Part print with two shaded views. Sizes in mm from the minimum x, y, z corner. A direction names the side the tool comes from. Round coordinates to 2 decimals unless told otherwise and drop trailing zeros. Write each loop counter-clockwise with the first axis right and the second up, starting at its lowest first coordinate (ties: lowest second). Pieces come first, ordered by that corner, then holes. Notation, with made-up numbers: (72, 29) - (86, 29) arc R16 cw to (86, 38) - close; hole circle Ø4 at (63, 0.5). An arc over 180 degrees is marked (long way). Answer as a JSON object with one key per item and string values. Group by question number.
Item 1: Flat gauge pin, fed straight in: pin 1 (3.5 mm diameter, centred on x = 3.5, y = 4.5, fed in from -Z). Where does the tip first touch, or does it go through?
Item 2: Two-plate mould, pull along Z, no slides. Class the marked faces 4, 5 and 6: +Z half, -Z half, draft (parallel to the pull), parting line (faces both ways), or undercut.
Item 3: Which spindle directions (+Z, -Z, +X, -X, +Y, -Y) get a long thin tool onto all of the face, cutting with end or side? Do the marked faces 1, 2 and 3. Say none if no direction does.
Item 4: Slice it at C-C, the plane z = 1.25. List the corners of the cut face in (x, y).
Item 5: Slice it at D-D, the plane x = 1.75. List the corners of the cut face in (y, z), then the cut area to 3 significant figures.
Item 6: Slice it at B-B, the plane x = 9. Give the number of separate pieces and of enclosed holes in the cut face.
Item 7: Probe line 1 (Z direction, x = 4, y = 4); line 2 (Y direction, x = 8.5, z = 2) (1 decimal); line 3 (Z direction, x = 8.5, y = 10.75). List the from-to ranges inside material, lowest first. Write a range as from..to.
Item 8: Slice it at A-A, the plane z = 5.5. List the corners of the cut face in (x, y).
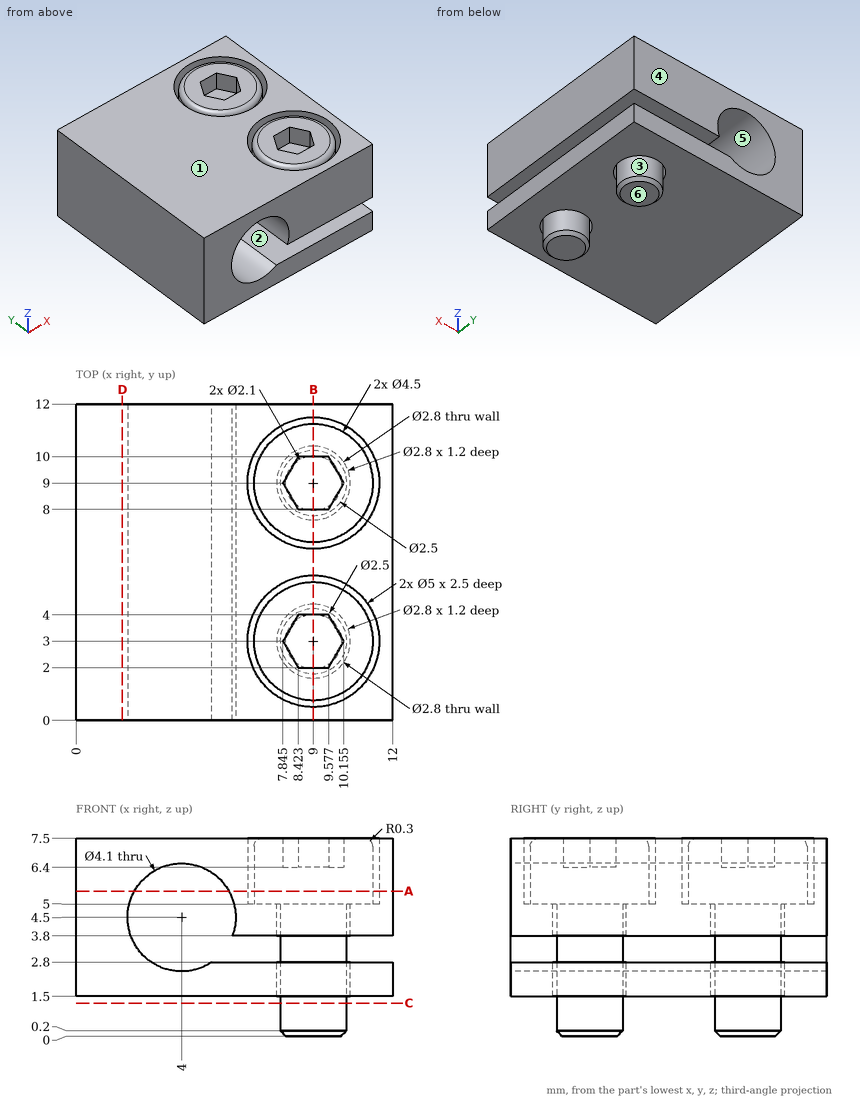
Geometry says:
{
 "1": {"pin 1": "stops at z = 1.5"},
 "2": {"face 4": "draft", "face 5": "undercut", "face 6": "-Z half"},
 "3": {"face 1": "+Z, +X, -X, +Y, -Y", "face 2": "none", "face 3": "-Z"},
 "4": {"outline": "circle Ø2.5 at (9, 3); circle Ø2.5 at (9, 9)"},
 "5": {"outline": "(0, 1.5) - (12, 1.5) - (12, 7.5) - (0, 7.5) - close", "area": "72.0 mm^2"},
 "6": {"separate pieces": "4", "enclosed holes": "0"},
 "7": {"line 1": "z = 1.5..2.45, 6.55..7.5", "line 2": "y = 0..1.7, 1.9..4.1, 4.3..7.7, 7.9..10.1, 10.3..12", "line 3": "z = 1.5..2.8, 3.8..7.5"},
 "8": {"outline": "(0, 0) - (2.21, 0) - (2.21, 12) - (0, 12) - close; (5.79, 0) - (12, 0) - (12, 12) - (5.79, 12) - close; circle Ø4.5 at (9, 3); circle Ø4.5 at (9, 9); hole circle Ø5 at (9, 3); hole circle Ø5 at (9, 9)"}
}
